from build123d import *

# Parameters (mm, degrees)
SKETCH1_R           = 150
BOSS_EXTRUDE1_DEPTH = 35
SKETCH2_R           = 4
CUT_EXTRUDE1_DEPTH  = 30
SKETCH3_R           = 8
SKETCH3_R_2         = 46.138899257
CUT_EXTRUDE2_DEPTH  = 5
FILLET1_R           = 10


with BuildPart() as part:
    # Sketch1 → Boss-Extrude1 (new body)
    with BuildSketch(Plane(origin=(0, 0, 0), x_dir=(1, 0, 0), z_dir=(0, 1, 0))):
        with Locations(Location((0, 0, 0), (0, 0, 270))):
            Circle(SKETCH1_R)
    extrude(amount=BOSS_EXTRUDE1_DEPTH)

    # Sketch2 → Cut-Extrude1 (cut)
    with BuildSketch(Plane.XZ):
        with Locations(Location((0, 52, 0), (0, 0, 270))):
            Circle(SKETCH2_R)
        with Locations(Location((-52, 0, 0), (0, 0, 270))):
            Circle(SKETCH2_R)
        with Locations(Location((52, 0, 0), (0, 0, 270))):
            Circle(SKETCH2_R)
        with Locations(Location((0, -52, 0), (0, 0, 270))):
            Circle(SKETCH2_R)
    extrude(amount=-CUT_EXTRUDE1_DEPTH, mode=Mode.SUBTRACT)

    # Sketch3 → Cut-Extrude2 (cut)
    with BuildSketch(Plane(origin=(0, 35, 0), x_dir=(1, 0, 0), z_dir=(0, 1, 0))):
        with BuildLine():
            ThreePointArc((-52, 8), (-60, 0), (-52, -8))
            ThreePointArc((-52, -8), (-48.606472063, -7.244581985), (-45.85382716, -5.120992035))
            ThreePointArc((-45.85382716, -5.120992035), (-46.138899257, 0), (-45.85382716, 5.120992035))
            ThreePointArc((-45.85382716, 5.120992035), (-48.606472063, 7.244581985), (-52, 8))
        make_face()
        with BuildLine():
            Line((-52, -8), (-45.440048687, -8))
            ThreePointArc((-45.440048687, -8), (-45.669630101, -6.563757396), (-45.85382716, -5.120992035))
            ThreePointArc((-45.85382716, -5.120992035), (-48.606472063, -7.244581985), (-52, -8))
        make_face()
        with BuildLine():
            Line((-45.440048687, 8), (-52, 8))
            ThreePointArc((-52, 8), (-48.606472063, 7.244581985), (-45.85382716, 5.120992035))
            ThreePointArc((-45.85382716, 5.120992035), (-45.669630101, 6.563757396), (-45.440048687, 8))
        make_face()
        with Locations((0, 52)):
            Circle(SKETCH3_R)
        Circle(SKETCH3_R_2)
        with Locations((-52, 0)):
            Circle(SKETCH3_R)
        with Locations((0, -52)):
            Circle(SKETCH3_R)
        with Locations((52, 0)):
            Circle(SKETCH3_R)
        with BuildLine():
            ThreePointArc((5.120992035, 45.85382716), (7.244581985, 48.606472063), (8, 52))
            ThreePointArc((8, 52), (0, 60), (-8, 52))
            ThreePointArc((-8, 52), (-7.244581985, 48.606472063), (-5.120992035, 45.85382716))
            ThreePointArc((-5.120992035, 45.85382716), (0, 46.138899257), (5.120992035, 45.85382716))
        make_face()
        with BuildLine():
            ThreePointArc((5.120992035, 45.85382716), (6.563757396, 45.669630101), (8, 45.440048687))
            Line((8, 45.440048687), (8, 52))
            ThreePointArc((8, 52), (7.244581985, 48.606472063), (5.120992035, 45.85382716))
        make_face()
        with BuildLine():
            ThreePointArc((-5.120992035, 45.85382716), (-7.244581985, 48.606472063), (-8, 52))
            Line((-8, 52), (-8, 45.440048687))
            ThreePointArc((-8, 45.440048687), (-6.563757396, 45.669630101), (-5.120992035, 45.85382716))
        make_face()
        with BuildLine():
            ThreePointArc((45.85382716, -5.120992035), (48.606472063, -7.244581985), (52, -8))
            ThreePointArc((52, -8), (57.656854249, -5.656854249), (60, 0))
            ThreePointArc((60, 0), (57.656854249, 5.656854249), (52, 8))
            ThreePointArc((52, 8), (48.606472063, 7.244581985), (45.85382716, 5.120992035))
            ThreePointArc((45.85382716, 5.120992035), (46.067576106, 2.564460252), (46.138899257, 0))
            ThreePointArc((46.138899257, 0), (46.067576106, -2.564460252), (45.85382716, -5.120992035))
        make_face()
        with BuildLine():
            Line((45.440048687, -8), (52, -8))
            ThreePointArc((52, -8), (48.606472063, -7.244581985), (45.85382716, -5.120992035))
            ThreePointArc((45.85382716, -5.120992035), (45.669630101, -6.563757396), (45.440048687, -8))
        make_face()
        with BuildLine():
            ThreePointArc((45.85382716, 5.120992035), (48.606472063, 7.244581985), (52, 8))
            Line((52, 8), (45.440048687, 8))
            ThreePointArc((45.440048687, 8), (45.669630101, 6.563757396), (45.85382716, 5.120992035))
        make_face()
        with BuildLine():
            ThreePointArc((-8, -52), (0, -60), (8, -52))
            ThreePointArc((8, -52), (7.244581985, -48.606472063), (5.120992035, -45.85382716))
            ThreePointArc((5.120992035, -45.85382716), (0, -46.138899257), (-5.120992035, -45.85382716))
            ThreePointArc((-5.120992035, -45.85382716), (-7.244581985, -48.606472063), (-8, -52))
        make_face()
        with BuildLine():
            Line((-8, -45.440048687), (-8, -52))
            ThreePointArc((-8, -52), (-7.244581985, -48.606472063), (-5.120992035, -45.85382716))
            ThreePointArc((-5.120992035, -45.85382716), (-6.563757396, -45.669630101), (-8, -45.440048687))
        make_face()
        with BuildLine():
            Line((8, -52), (8, -45.440048687))
            ThreePointArc((8, -45.440048687), (6.563757396, -45.669630101), (5.120992035, -45.85382716))
            ThreePointArc((5.120992035, -45.85382716), (7.244581985, -48.606472063), (8, -52))
        make_face()
    extrude(amount=-CUT_EXTRUDE2_DEPTH, mode=Mode.SUBTRACT)

    # Fillet1
    fillet1_edges = [part.edges().sort_by_distance(p)[0] for p in [
        (-45.440048687, 32.5, 8),
        (-8, 32.5, 45.440048687),
        (8, 32.5, 45.440048687),
        (45.440048687, 32.5, 8),
        (45.440048687, 32.5, -8),
        (8, 32.5, -45.440048687),
        (-8, 32.5, -45.440048687),
        (-45.440048687, 32.5, -8),
    ]]
    fillet(fillet1_edges, radius=FILLET1_R)


solid = part.part
Verification items for the finished model (mm, model axes). A direction names the side the tool comes from. Give positions to 0.01 mm unless a question says otherwise; leave off trailing zeros. Write each loop counter-clockwise with the first axis right and the second up, starting at its lowest first coordinate (ties: lowest second). Pieces come first, ordered by that corner, then holes. Notation, with made-up numbers: (-12, -15.5) - (18, -15.5) arc R11 ccw to (18, -1.5) - close; hole circle Ø3 at (54, -6). An arc over 180 degrees is marked (long way). Answer as CSV lines item,"result". Start each with the question number.
1. Sectioned sample at D-D (x = 85). Record the boundary of the cut face in (y, z), then the cut area to 3 significant figures.
2. Draft check along Z on faces 3 (the face through (-1, 30, -1)), 4 (the face through (-91.273, 17.255, -119.035)), 5 (the face through (2, 0, -2)). Enter one of: pulls with the +Z half, pulls with the -Z half, needs draft (parallel to the pull), parting line crosses it, or undercut.
3. Sectioned sample at C-C (z = -34). Record the boundary of the cut face in (x, y).
4. Sectioned sample at B-B (y = 6). Record the boundary of the cut face in (x, z), then the cut area to 3 significant figures.
5. Depth check by flat-ended pin: pin 1 (5 mm diameter, centred on x = -1.5, y = 30, fed in from +Z); pin 2 (8 mm diameter, centred on y = 4.5, z = -105.5, fed in from +X); pin 3 (2 mm diameter, centred on y = 9, z = -2.5, fed in from -X); pin 4 (2 mm diameter, centred on y = 7, z = -85.5, fed in from -X). Enter the tip coordinate at first touch or a pass-through.
6. Sectioned sample at A-A (x = 0). Record the boundary of the cut face in (y, z).
7. Thickness scan on line 1 (X direction, y = 16.5, z = 0); line 2 (X direction, y = 9.75, z = -52); line 3 (X direction, y = 27, z = 55). Record the ranges inside material, lowest first.
8. Set-up check for faces 1 (the face through (0, 33, -60)), 2 (the face through (-1.532, 14.79, -55.695)): record each of +Z, -Z, +X, -X, +Y, -Y from which the full face is reachable in a straight line by a thin tool's end or side.
Derived:
1,outline,"(0, -123.59) - (35, -123.59) - (35, 123.59) - (0, 123.59) - close"
1,area,"8,650 mm²"
2,face 3,"undercut"
2,face 4,"parting line crosses it"
2,face 5,"needs draft"
3,outline,"(-146.1, 0) - (146.1, 0) - (146.1, 35) - (31.19, 35) - (31.19, 30) - (-31.19, 30) - (-31.19, 35) - (-146.1, 35) - close"
4,outline,"circle Ø300 at (0, 0); hole circle Ø8 at (-52, 0); hole circle Ø8 at (0, -52); hole circle Ø8 at (0, 52); hole circle Ø8 at (52, 0)"
4,area,"70,500 mm²"
5,pin 1,"z = 150"
5,pin 2,"x = 110.44"
5,pin 3,"x = -149.99"
5,pin 4,"x = -123.93"
6,outline,"(0, -150) - (35, -150) - (35, -60) - (30, -60) - (30, -56) - (0, -56) - close; (0, -48) - (30, -48) - (30, 48) - (0, 48) - close; (0, 56) - (30, 56) - (30, 60) - (35, 60) - (35, 150) - (0, 150) - close"
7,line 1,"-150 to -56, -48 to 48, 56 to 150"
7,line 2,"-140.7 to -4, 4 to 140.7"
7,line 3,"-139.55 to -2.65, 2.65 to 139.55"
8,face 1,"+Y"
8,face 2,"+Y, -Y"
